Could you check a few things on this drawing? It's one solid part, dimensions in mm from its lowest x, y, z. A direction names the side the tool comes from. Coordinates: 2 decimals unless noted, no trailing zeros. Write each loop counter-clockwise with the first axis right and the second up, starting at its lowest first coordinate (ties: lowest second). Pieces come first, ordered by that corner, then holes. Notation, with made-up numbers: (-22, 85.5) - (37, 85.5) arc R26 cw to (37, 103.5) - close; hole circle Ø2 at (22, 77.5). An arc over 180 degrees is marked (long way). Answer as a JSON object with one key per item and string values. Group by question number.
1) On a 3-axis mill with a long thin cutter (end or side, diameter ignored), from which of +Z, -Z, +X, -X, +Y, -Y can I reach the whole of each face in a straight line? I mean the marked faces 4 and 5. Say none if no direction works.
2) If we section it at A-A (z = 58.5): Write out the boundary of the cut face in (x, y) (1 decimal).
3) We'd pull the mould along X, two halves only. Please class the marked faces 1, 2 and 3: released by +X, released by -X, zero draft, split by the parting line, or undercut.
4) If we section it at C-C (x = 41): Write out the boundary of the cut face in (y, z).
5) Please list where these lines run through material, in increasing order: line 1 along X through (y, z) = (60.5, 60) (1 decimal); line 2 along Y through (x, z) = (10.5, 7.5).
6) If we section it at D-D (z = 35): Write out the boundary of the cut face in (x, y) (1 decimal), plus the area to 3 significant figures.
7) If we section it at B-B (y = 9): Write out the boundary of the cut face in (x, z) (1 decimal).
8) Will these pins go through, and if not, where does the flat tip stop? pin 1 Ø1 at (y, z) = (35, 29.5) entering from +X; pin 2 Ø0.8 at (x, y) = (33.5, 1.5) entering from +Z.
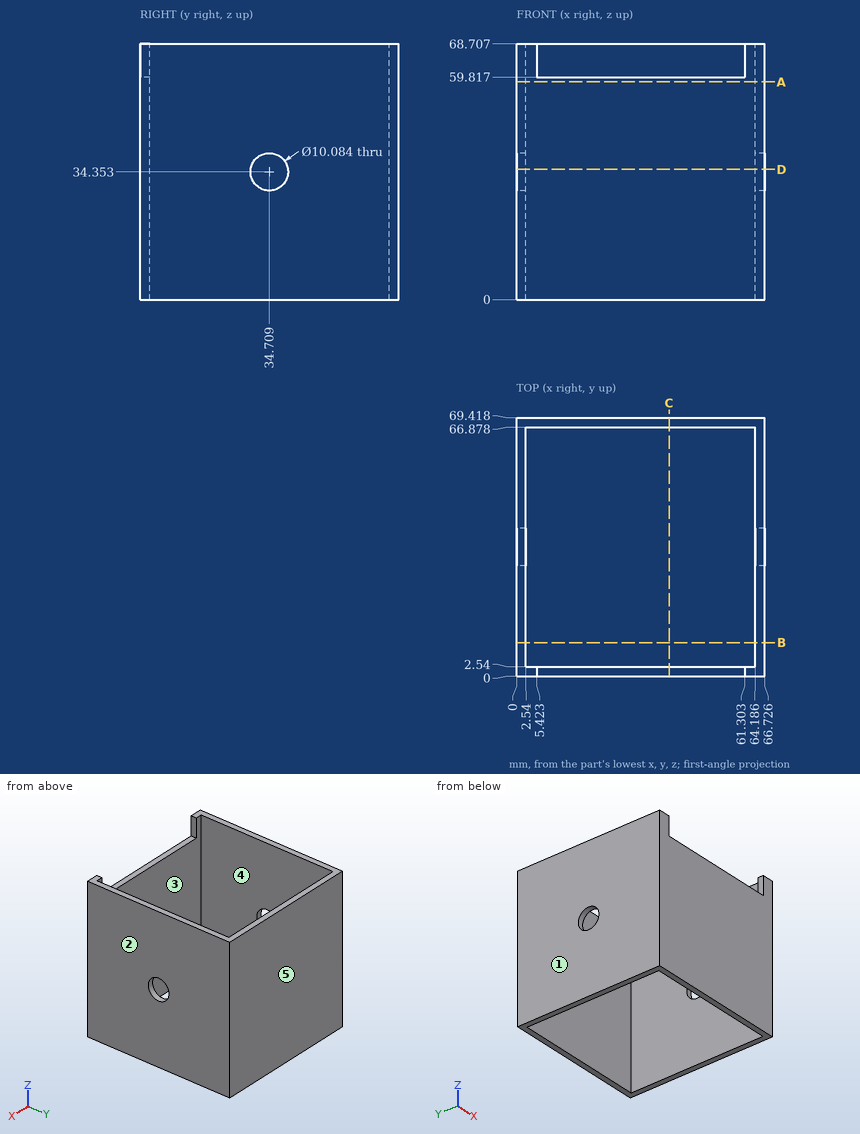
Here are the results:
{
 "1": {"face 4": "+Z, -Z", "face 5": "+Z, -Z, +X, -X, +Y"},
 "2": {"outline": "(0, 0) - (66.7, 0) - (66.7, 69.4) - (0, 69.4) - close; hole (2.5, 2.5) - (64.2, 2.5) - (64.2, 66.9) - (2.5, 66.9) - close"},
 "3": {"face 1": "released by -X", "face 2": "released by +X", "face 3": "undercut"},
 "4": {"outline": "(0, 0) - (2.54, 0) - (2.54, 59.82) - (0, 59.82) - close; (66.88, 0) - (69.42, 0) - (69.42, 68.71) - (66.88, 68.71) - close"},
 "5": {"line 1": "x = 0 to 2.5, 64.2 to 66.7", "line 2": "y = 0 to 2.54, 66.88 to 69.42"},
 "6": {"outline": "(0, 0) - (66.7, 0) - (66.7, 29.7) - (64.2, 29.7) - (64.2, 2.5) - (2.5, 2.5) - (2.5, 29.7) - (0, 29.7) - close; (0, 39.7) - (2.5, 39.7) - (2.5, 66.9) - (64.2, 66.9) - (64.2, 39.7) - (66.7, 39.7) - (66.7, 69.4) - (0, 69.4) - close", "area": "615 mm²"},
 "7": {"outline": "(0, 0) - (2.5, 0) - (2.5, 68.7) - (0, 68.7) - close; (64.2, 0) - (66.7, 0) - (66.7, 68.7) - (64.2, 68.7) - close"},
 "8": {"pin 1": "stops at x = 66.73", "pin 2": "stops at z = 59.82"}
}
